from build123d import *

# Parameters (mm, degrees)
SKETCH_1_W      = 25
SKETCH_1_H      = 23.5
SKETCH_1_R      = 1.5
EXTRUDE_1_DEPTH = 4
SKETCH_2_W      = 30
SKETCH_2_H      = 23.5
SKETCH_2_R      = 1.5
EXTRUDE_2_DEPTH = 4
CHAMFER_1_SIZE  = 2
FILLET_1_R      = 1


with BuildPart() as part:
    # 草图1 → 凸台-拉伸1 (new body)
    with BuildSketch(Plane.XY):
        with Locations((2.963131814, 3.167575845)):
            Rectangle(SKETCH_1_W, SKETCH_1_H)
        with Locations((2.463131814, 10.917575845)):
            Circle(SKETCH_1_R, mode=Mode.SUBTRACT)
        with Locations((-5.536868186, -4.582424155)):
            Circle(SKETCH_1_R, mode=Mode.SUBTRACT)
        with Locations((9.463131814, -4.582424155)):
            Circle(SKETCH_1_R, mode=Mode.SUBTRACT)
    extrude(amount=EXTRUDE_1_DEPTH)

    # 草图2 → 凸台-拉伸2 (add)
    with BuildSketch(Plane(origin=(15.463131814, 0, 0), x_dir=(0, 0, -1), z_dir=(1, 0, 0))):
        with Locations((11, 3.167575845)):
            Rectangle(SKETCH_2_W, SKETCH_2_H)
        with Locations(Location((6, 10.417575845, 0), (0, 0, 90))):
            Circle(SKETCH_2_R, mode=Mode.SUBTRACT)
        with Locations(Location((21, 10.417575845, 0), (0, 0, 90))):
            Circle(SKETCH_2_R, mode=Mode.SUBTRACT)
        with Locations(Location((6, -4.582424155, 0), (0, 0, 90))):
            Circle(SKETCH_2_R, mode=Mode.SUBTRACT)
        with Locations(Location((21, -4.582424155, 0), (0, 0, 90))):
            Circle(SKETCH_2_R, mode=Mode.SUBTRACT)
    extrude(amount=EXTRUDE_2_DEPTH)

    # 倒角1
    chamfer_1_edges = [part.edges().sort_by_distance(p)[0] for p in [
        (15.463131814, 3.167575845, 0),
    ]]
    chamfer(chamfer_1_edges, length=CHAMFER_1_SIZE)

    # 圆角1
    fillet_1_edges = [part.edges().sort_by_distance(p)[0] for p in [
        (4.963131814, 14.917575845, 4),
        (19.463131814, 3.167575845, 4),
        (19.463131814, -8.582424155, -11),
        (19.463131814, 3.167575845, -26),
        (19.463131814, 14.917575845, -11),
        (15.463131814, 3.167575845, -26),
        (17.463131814, -8.582424155, -26),
        (15.463131814, 14.917575845, -14),
        (17.463131814, 14.917575845, -26),
        (15.463131814, -8.582424155, -14),
        (15.463131814, 3.167575845, -2),
        (1.963131814, 14.917575845, 0),
        (-9.536868186, 3.167575845, 4),
        (13.463131814, 3.167575845, 0),
        (14.463131814, 14.917575845, -1),
        (14.463131814, -8.582424155, -1),
        (1.963131814, -8.582424155, 0),
        (-9.536868186, 3.167575845, 0),
        (-9.536868186, 14.917575845, 2),
        (-9.536868186, -8.582424155, 2),
        (4.963131814, -8.582424155, 4),
    ]]
    fillet(fillet_1_edges, radius=FILLET_1_R)


solid = part.part
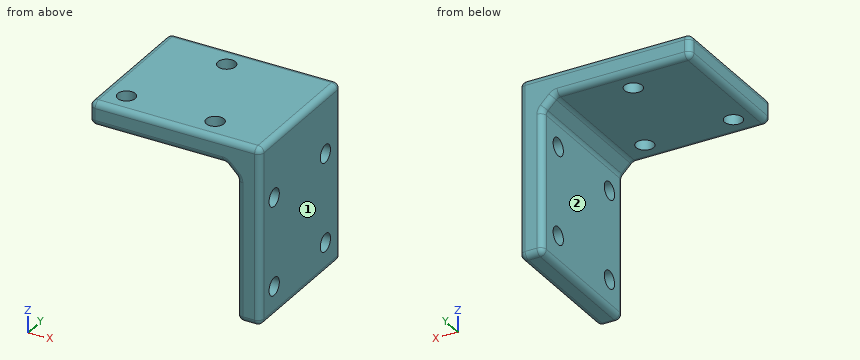
Can you work these out from the model? Positions are in its coordinate system, mm. Face numbers are marked on the shaded views. A direction names the side the tool comes from. Give positions to 0.01 mm unless a question says otherwise; leave off trailing zeros. Order: outer loops, then holes, each group sorted by start corner. A loop starts at its lowest first (then second) coordinate and runs counter-clockwise, first axis right, second up. Notation, with made-up numbers: M 5,0 L 50,0 A11 cw 50,15 Z; hole C -3,-1 d10. An arc over 180 degrees is marked long. Use a Markdown table: item, result. Add a question column.
Item 1: Will these pins go through, and if not, where does the flat tip stop? pin 1 (2 mm diameter, centred on y = 5.5, z = -6.5, fed in from -X); pin 2 (4 mm diameter, centred on x = 11.5, y = 0, fed in from -Z); pin 3 (5 mm diameter, centred on x = 5, y = 4.5, fed in from -Z).
Item 2: If I drill on L1, parallel to Z at x = 3.25, y = -3.25; L2, parallel to X at y = 7.5, z = -4.5; L3, parallel to X at y = 12, z = 0.25, over which ranges is the centre line in solid material (lowest first)? Write a range as [from, to].
Item 3: Suppose I cut it at C-C (x = 4.5). List the corners of the cut face in (y, z) for me, then the cut area to 3 significant figures.
Item 4: Suppose I cut it at D-D (y = 8.25). List the corners of the cut face in (x, z) for me.
Item 5: Suppose I cut it at B-B (z = -10.25). List the corners of the cut face in (x, y) for me.
Item 6: Suppose I cut it at A-A (z = -21). List the corners of the cut face in (x, y) for me, then the cut area to 3 significant figures.
Item 7: For the marked faces 1 and 2, which set-ups out of +Z, -Z, +X, -X, +Y, -Y let a thin tool reach every point of the face, with its end or its side?
Answer sheet:
| question | item | result |
|---|---|---|
| 1 | pin 1 | stops at x = 15.46 |
| 1 | pin 2 | stops at z = -0.11 |
| 1 | pin 3 | stops at z = 0 |
| 2 | L1 | z = [0, 4] |
| 2 | L2 | x = [15.46, 19.46] |
| 2 | L3 | x = [-9.2, 1.42], [3.5, 19.46] |
| 3 | outline | M -8.58,1 A1 ccw -7.58,0 L 13.92,0 A1 ccw 14.92,1 L 14.92,3 A1 ccw 13.92,4 L -7.58,4 A1 ccw -8.58,3 Z |
| 3 | area | 93.1 mm² |
| 4 | outline | M -9.54,1 A1 ccw -8.54,0 L 13.05,0 A1 cw 13.76,-0.29 L 15.17,-1.71 A1 cw 15.46,-2.41 L 15.46,-25 A1 ccw 16.46,-26 L 18.46,-26 A1 ccw 19.46,-25 L 19.46,3 A1 ccw 18.46,4 L -8.54,4 A1 ccw -9.54,3 Z |
| 5 | outline | M 15.46,-7.58 A1 ccw 16.46,-8.58 L 18.46,-8.58 A1 ccw 19.46,-7.58 L 19.46,13.92 A1 ccw 18.46,14.92 L 16.46,14.92 A1 ccw 15.46,13.92 Z |
| 6 | outline | M 15.46,-7.58 A1 ccw 16.46,-8.58 L 18.46,-8.58 A1 ccw 19.46,-7.58 L 19.46,-6.08 L 15.46,-6.08 Z; M 15.46,-3.08 L 19.46,-3.08 L 19.46,8.92 L 15.46,8.92 Z; M 15.46,11.92 L 19.46,11.92 L 19.46,13.92 A1 ccw 18.46,14.92 L 16.46,14.92 A1 ccw 15.46,13.92 Z |
| 6 | area | 69.1 mm² |
| 7 | face 1 | +Z, -Z, +X, +Y, -Y |
| 7 | face 2 | -Z, -X, +Y, -Y |
